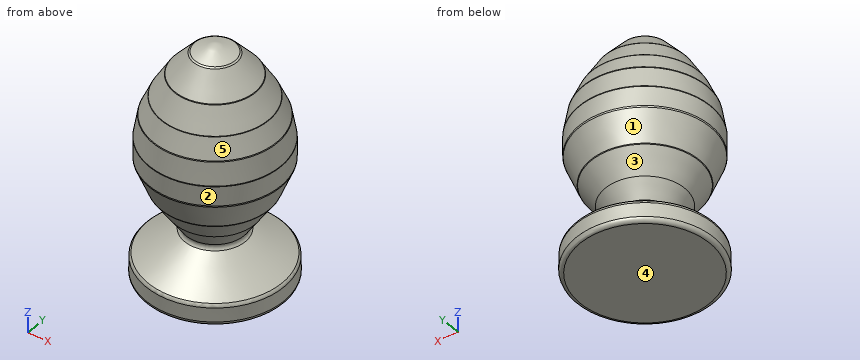
```python
from build123d import *

# Parameters (mm, degrees)
F2_R = 5.08


with BuildPart() as f1:
    # F0 (on Front) → F1 (revolve)
    with BuildSketch(Plane.XZ):
        Polygon((26.503066, 283.759713), (0, 294.11453), (0, 0), (87.615736, 0), (87.39959, 25.638381), (34.229953, 61.084811), (50.386176, 85.670367), (68.649732, 113.065697), (83.401062, 149.592802), (83.401062, 175.583258), (78.483954, 203.681022), (67.947291, 227.564156), (51.08862, 255.661905), align=None)
    revolve(axis=Axis((0, 0, 147.057265), (0, 0, -1)))

    # F2
    f2_edges = [f1.edges().sort_by_distance(p)[0] for p in [
        (-51.08862, 0, 255.661905),
        (-67.947291, 0, 227.564156),
        (-83.401062, 0, 175.583258),
        (-78.483954, 0, 203.681022),
        (-83.401062, 0, 149.592802),
        (-26.503066, 0, 283.759713),
        (-68.649732, 0, 113.065697),
        (-50.386176, 0, 85.670367),
        (-34.229953, 0, 61.084811),
        (-87.39959, 0, 25.638381),
        (-87.615736, 0, 0),
    ]]
    fillet(f2_edges, radius=F2_R)


solid = f1.part
```
Build history of the part. All positions in model axes, mm. Face numbers are marked on the shaded views. A direction names the side the tool comes from. Round coordinates to 2 decimals unless told otherwise and drop trailing zeros. Write each loop counter-clockwise with the first axis right and the second up, starting at its lowest first coordinate (ties: lowest second). Pieces come first, ordered by that corner, then holes. Notation, with made-up numbers: (64, 13) - (68, 13) arc R20 cw to (68, 45) - close; hole circle Ø2 at (71, 42). An arc over 180 degrees is marked (long way). Write each question's results on one line, items separated by ' | '. Start each with the question number.
Item 1: Drop flat-ended pins along their axis: P1, Ø6, axis at x = 47.5, y = -18, coming from the +Z side; P2, Ø12, axis at y = 20, z = 210, coming from the +X side; P3, Ø10, axis at y = 59, z = 52.5, coming from the -X side; P4, Ø12, axis at x = 2, y = -59, coming from the +Z side. Give the stop position or say it passes through.
Item 2: Mould opens along Z. For the marked faces 3, 4 and 5 say: pulls with the +Z half, pulls with the -Z half, needs draft (parallel to the pull), parting line crosses it, or undercut.
Item 3: Wall check: L1, parallel to Z at x = -22, y = -39.5; L2, parallel to Z at x = -8, y = 66.5; L3, parallel to X at y = 17.5, z = 117. Give the ranges that are in metal, low to high. Write a range as [from, to].
Item 4: Saw through at B-B (z = 252). Write the cut outline in (x, y), and give its area (3 significant figures).
Item 5: Which spindle directions (+Z, -Z, +X, -X, +Y, -Y) get a long thin tool onto all of the face, cutting with end or side? Do the marked faces 1 and 2. Say none if no direction does.
Item 6: Saw through at A-A (z = 19). Write the cut outline in (x, y).
Results are:
1) P1: stops at z = 259.42 | P2: stops at x = 76.12 | P3: passes through | P4: stops at z = 252.42
2) face 3: undercut | face 4: pulls with the -Z half | face 5: pulls with the +Z half
3) L1: z = [0, 53.76], [77.8, 262.38] | L2: z = [0, 39.25], [110.56, 229.18] | L3: x = [-68.02, 68.02]
4) outline: circle Ø106.57 at (0, 0) | area: 8,920 mm²
5) face 1: none | face 2: +Z
6) outline: circle Ø174.91 at (0, 0)
